from build123d import *

# Parameters (mm, degrees)
SM_BASE_FLANGE_1_DEPTH = 25
SKETCH_6_W             = 3.75
SKETCH_6_H             = 2
SKETCH_6_W_2           = 15
CUT_EXTRUDE_1_DEPTH    = 10
SKETCH_7_R             = 0.75
EXTRUDE_1_DEPTH        = 2


# Sheet-metal steps are written as plain solids
with BuildPart() as part:
    # Sketch 2 → 基体-法兰1 (new body)
    with BuildSketch(Plane.XY):
        with BuildLine():
            Line((4.25, -6.75), (4.25, 0))
            ThreePointArc((4.25, 0), (0, 4.25), (-4.25, 0))
            Line((-4.25, 0), (-4.25, -6.75))
            Line((-4.25, -6.75), (-2.75, -6.75))
            Line((-2.75, -6.75), (-2.75, 0))
            ThreePointArc((-2.75, 0), (0, 2.75), (2.75, 0))
            Line((2.75, 0), (2.75, -6.75))
            Line((2.75, -6.75), (4.25, -6.75))
        make_face()
    extrude(amount=SM_BASE_FLANGE_1_DEPTH)

    # 草图6 → 切除-拉伸1 (cut)
    with BuildSketch(Plane.ZY.offset(4.25)):
        with Locations((1.875, -5.75)):
            Rectangle(SKETCH_6_W, SKETCH_6_H)
        with Locations((12.75, -5.75)):
            Rectangle(SKETCH_6_W_2, SKETCH_6_H)
        with Locations((23.125, -5.75)):
            Rectangle(SKETCH_6_W, SKETCH_6_H)
    extrude(amount=-CUT_EXTRUDE_1_DEPTH, mode=Mode.SUBTRACT)

    # 草图7 → 凸台-拉伸1 (add)
    with BuildSketch(Plane.XZ.offset(4.75)):
        with Locations((-3.5, 20)):
            Circle(SKETCH_7_R)
        with Locations((-3.5, 5.5)):
            Circle(SKETCH_7_R)
        with Locations((3.5, 5.5)):
            Circle(SKETCH_7_R)
        with Locations((3.5, 20)):
            Circle(SKETCH_7_R)
    extrude(amount=EXTRUDE_1_DEPTH)


solid = part.part
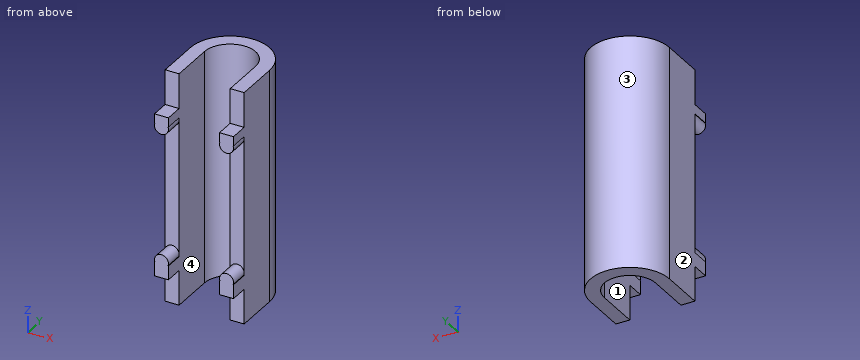
Check sheet for the modelled part. Datum: model origin and axes. Units: mm. Face numbers are marked on the shaded views. Give positions to 0.01 mm unless a question says otherwise; leave off trailing zeros. Write each loop counter-clockwise with the first axis right and the second up, starting at its lowest first coordinate (ties: lowest second). Pieces come first, ordered by that corner, then holes. Notation, with made-up numbers: (-17.75, 17.25) -> (-2.75, 17.25) arc R26 cw to (-2.75, 33.25) -> close; hole circle Ø9 at (6, 36). An arc over 180 degrees is marked (long way). One line per item, written item: value. Start each with the question number.
Item 1: Material ranges on probe 1 along X at (y, z) = (-2.5, 21.75); probe 2 along X at (y, z) = (1, 2); probe 3 along Y at (x, z) = (2.25, 14.25), recorded low to high. Write a range as from..to.
Item 2: Section check D-D on y = 3.75. Record the cut outline in (x, z), then the cut area to 4 significant figures.
Item 3: Gauge pin test, flat ends, axial feed: pin 1 (0.8 mm diameter, centred on x = -3.5, z = 24, fed in from -Y); pin 2 (1.2 mm diameter, centred on x = 3.5, y = -6, fed in from -Z); pin 3 (1.5 mm diameter, centred on y = 2.5, z = 9, fed in from -X). Record the tip position at first contact, or that the pin passes through.
Item 4: Draft check along X on the marked faces 1, 2, 3 and 4. Enter one of: +X half, -X half, draft (parallel to the pull), parting line (faces both ways), or undercut.
Item 5: Section check C-C on x = 0. Record the cut outline in (y, z), then the cut area to 3 significant figures.
Item 6: Section check A-A on y = -2. Record the cut outline in (x, z).
Item 7: Section check B-B on z = 19.75. Record the cut outline in (x, y).
Results list:
1. probe 1: -4.25..-2.75, 2.75..4.25
1. probe 2: -4.13..-2.56, 2.56..4.13
1. probe 3: 1.58..3.61
2. outline: (-2, 0) -> (2, 0) -> (2, 25) -> (-2, 25) -> close
2. area: 100.0 mm²
3. pin 1: y = -4.75
3. pin 2: z = 3.75
3. pin 3: x = -3.87
4. face 1: undercut
4. face 2: -X half
4. face 3: parting line
4. face 4: undercut
5. outline: (2.75, 0) -> (4.25, 0) -> (4.25, 25) -> (2.75, 25) -> close
5. area: 37.5 mm²
6. outline: (-4.25, 0) -> (-2.75, 0) -> (-2.75, 25) -> (-4.25, 25) -> close; (2.75, 0) -> (4.25, 0) -> (4.25, 25) -> (2.75, 25) -> close
7. outline: (-4.25, -4.75) -> (-4.21, -4.75) -> (-4.21, -6.75) -> (-2.79, -6.75) -> (-2.79, -4.75) -> (-2.75, -4.75) -> (-2.75, 0) arc R2.75 cw to (2.75, 0) -> (2.75, -4.75) -> (2.79, -4.75) -> (2.79, -6.75) -> (4.21, -6.75) -> (4.21, -4.75) -> (4.25, -4.75) -> (4.25, 0) arc R4.25 ccw to (-4.25, 0) -> close
